Model file for the job. Use its own axes, mm. Coordinates: 2 decimals unless noted, no trailing zeros. Order: outer loops, then holes, each group sorted by start corner. A loop starts at its lowest first (then second) coordinate and runs counter-clockwise, first axis right, second up. Notation, with made-up numbers: M 41,60.25 L 65,60.25 A36 ccw 65,95.25 Z; hole C 61.5,19.25 d1. An arc over 180 degrees is marked long. Return JSON: item names as keys, results as strings.
```python
from build123d import *

# Parameters (mm, degrees)
F0_W     = 2400
F0_H     = 600
F0_W_2   = 2300
F0_H_2   = 500
F1_DEPTH = 100
F2_R     = 4
F3_DEPTH = 50
F4_R     = 4
F5_DEPTH = 50


with BuildPart() as f1:
    # F0 (on Top) → F1 (new body)
    with BuildSketch(Plane.XY):
        Rectangle(F0_W, F0_H)
        Rectangle(F0_W_2, F0_H_2, mode=Mode.SUBTRACT)
    extrude(amount=F1_DEPTH)

    # F2 (on face) → F3 (cut, through all)
    with BuildSketch(Plane.XZ.offset(-250)):
        with Locations((810, 32)):
            Circle(F2_R)
        with Locations((1050, 68)):
            Circle(F2_R)
    extrude(amount=-F3_DEPTH, mode=Mode.SUBTRACT)

    # F4 (on face) → F5 (cut, through all)
    with BuildSketch(Plane(origin=(0, -250, 0), x_dir=(-1, 0, 0), z_dir=(0, 1, 0))):
        with Locations((-810, 32)):
            Circle(F4_R)
        with Locations((-1050, 68)):
            Circle(F4_R)
    extrude(amount=-F5_DEPTH, mode=Mode.SUBTRACT)


solid = f1.part
```
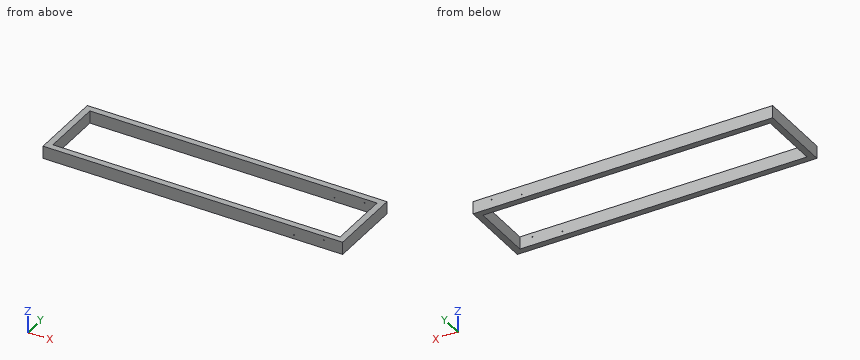
Item 1: Saw through at B-B (x = -16). Write the cut outline in (y, z).
Check result:
{"outline": "M -300,0 L -250,0 L -250,100 L -300,100 Z; M 250,0 L 300,0 L 300,100 L 250,100 Z"}
Item 2: Wall check: line 1 (Y direction, x = 443.5, z = 39); line 2 (X direction, y = -155, z = 66.5); line 3 (Z direction, x = 810, y = -261.5). Give the ranges that are in metal, low to high.
Check result:
{"line 1": "y = -300 to -250, 250 to 300", "line 2": "x = -1200 to -1150, 1150 to 1200", "line 3": "z = 0 to 28, 36 to 100"}
Item 3: Saw through at A-A (y = -126). Write the cut outline in (x, z).
Check result:
{"outline": "M -1200,0 L -1150,0 L -1150,100 L -1200,100 Z; M 1150,0 L 1200,0 L 1200,100 L 1150,100 Z"}
